from build123d import *

# Parameters (mm, degrees)
F0_W     = 100
F0_H     = 200
F1_DEPTH = 10
F2_D     = 5
F3_D     = 4.2
F4_D     = 23
F5_D     = 5.5
F6_D     = 5.5
F7_D     = 5
F7_DEPTH = 15
F7_TIP   = 1.5021515476


with BuildPart() as f1:
    # F0 (on Right) → F1 (new body)
    with BuildSketch(Plane.YZ):
        Rectangle(F0_W, F0_H)
    extrude(amount=-F1_DEPTH)

    # F2 (through all)
    with Locations(Plane.YZ):
        with Locations((0, 39), (0, 87), (0, -39), (0, -87)):
            Hole(F2_D / 2)

    # F3 (through all)
    with Locations(Plane.YZ):
        with Locations((-23, -18), (-23, 0), (23, 0), (23, -18)):
            Hole(F3_D / 2)

    # F4 (through all)
    with Locations(Plane.YZ):
        with Locations((0, 0)):
            Hole(F4_D / 2)

    # F5 (through all)
    with Locations(Plane.YZ):
        with Locations((-40, 90), (-40, 70), (-40, 50), (-40, 30), (-40, -20), (-40, -40), (-40, -60), (-40, -80)):
            Hole(F5_D / 2)

    # F6 (through all)
    with Locations(Plane.YZ):
        with Locations((-40, -95), (-15, -95), (15, -95), (40, -95)):
            Hole(F6_D / 2)

    # F7
    with Locations(Plane.YZ):
        with Locations((34.75, 34.75), (-34.75, 34.75), (-34.75, -34.75), (34.75, -34.75)):
            Hole(F7_D / 2, depth=F7_DEPTH)
            with Locations((0, 0, -(F7_DEPTH + F7_TIP / 2))):  # 118° drill point
                Cone(0, F7_D / 2, F7_TIP, mode=Mode.SUBTRACT)


solid = f1.part
The model under review builds one solid part; all positions refer to its coordinate system, in mm. Round coordinates to 2 decimals unless told otherwise and drop trailing zeros. Write each loop counter-clockwise with the first axis right and the second up, starting at its lowest first coordinate (ties: lowest second). Pieces come first, ordered by that corner, then holes. Notation, with made-up numbers: (-24.75, 38) - (20.25, 38) arc R12 cw to (20.25, 50) - close; hole circle Ø7 at (2.25, -15.75). An arc over 180 degrees is marked (long way). One line per item, written item: value. Start each with the question number.
1. The part is to be moulded in two halves that separate along Z. For faces 1 (the face through (-10, -12, 1)), 2 (the face through (-5, -1, 100)), 3 (the face through (-5.07, -37.135, -33.999)), say which applies: released by +Z, released by -Z, zero draft, split by the parting line, or undercut.
2. Consider section D-D on y = 34.75. Write out the cut boundary in (x, z), and give its area (3 significant figures).
3. To check wall thickness, follow L1, parallel to Z at x = -7, y = 0; L2, parallel to Z at x = -2.25, y = -34.75; L3, parallel to Y at x = -7.5, z = 34.5. State the ranges of each line that lie inside material, in increasing order. Write a range as from..to.
4. Consider section B-B on x = -8. State how many separate pieces and enclosed holes the cut face has, and give its area (3 significant figures).
5. Consider section A-A on y = 23. Write out the cut boundary in (x, z), and give its area (3 significant figures).
6. Consider section C-C on y = 4.5. Write out the cut boundary in (x, z).
Checks:
1. face 1: zero draft
1. face 2: released by +Z
1. face 3: undercut
2. outline: (-10, -100) - (0, -100) - (0, -37.25) - (-10, -37.25) - close; (-10, -32.25) - (0, -32.25) - (0, 32.25) - (-10, 32.25) - close; (-10, 37.25) - (0, 37.25) - (0, 100) - (-10, 100) - close
2. area: 1,900 mm^2
3. L1: z = -100..-89.5, -84.5..-41.5, -36.5..-11.5, 11.5..36.5, 41.5..84.5, 89.5..100
3. L2: z = -100..-37.25, -32.25..32.25, 37.25..100
3. L3: y = -50..-37.24, -32.26..32.26, 37.24..50
4. separate pieces: 1
4. enclosed holes: 25
4. area: 19,100 mm^2
5. outline: (-10, -100) - (0, -100) - (0, -20.1) - (-10, -20.1) - close; (-10, -15.9) - (0, -15.9) - (0, -2.1) - (-10, -2.1) - close; (-10, 2.1) - (0, 2.1) - (0, 100) - (-10, 100) - close
5. area: 1,920 mm^2
6. outline: (-10, -100) - (0, -100) - (0, -10.58) - (-10, -10.58) - close; (-10, 10.58) - (0, 10.58) - (0, 100) - (-10, 100) - close
